Solid Edge part; units mm, degrees
sketch "Sketch1" plane through (0, 0, 0) normal (0, -1, 0) x (1, 0, 0)
  line L0 (2, 27.36) -> (2, 11.4867)
  line L1 (2, 11.4867) -> (4, 11.4867)
  line L2 (4, 11.4867) -> (4, 4.2309)
  line L3 (4, 4.2309) -> (7, 4.2309)
  line L4 (7, 4.2309) -> (7, 0)
  line L5 (7, 0) -> (1.25, 0)
  line L6 (1.25, 0) -> (1.25, 4.2309)
  line L7 (1.25, 27.36) -> (1.25, 4.2309)
  line L8 (1.25, 27.36) -> (2, 27.36)
revolve "RevolvedProtrusion1" add sketch "Sketch1" angle 360 about axis through (0, 0, 54) along (0, 0, -1)
cosmetic_thread "Thread1"
CAD build for the part. Positions are in the model's coordinates, mm. A direction names the side the tool comes from. Round coordinates to 2 decimals unless told otherwise and drop trailing zeros. Order: outer loops, then holes, each group sorted by start corner. A loop starts at its lowest first (then second) coordinate and runs counter-clockwise, first axis right, second up. Notation, with made-up numbers: (56.25, -1) -> (71.25, -1) arc R21 ccw to (71.25, 9) -> close; hole circle Ø8 at (-25.75, -33). An arc over 180 degrees is marked (long way). One line per question, with ' | ' between items.
Q1. Slice it at A-A (y = 0). Write the cut outline in (x, z), then the cut area to 3 significant figures.
Completed:
outline: (-7, 0) -> (-1.25, 0) -> (-1.25, 27.36) -> (-2, 27.36) -> (-2, 11.49) -> (-4, 11.49) -> (-4, 4.23) -> (-7, 4.23) -> close; (1.25, 0) -> (7, 0) -> (7, 4.23) -> (4, 4.23) -> (4, 11.49) -> (2, 11.49) -> (2, 27.36) -> (1.25, 27.36) -> close | area: 112 mm^2
Q2. Probe probe 1 along X at (y, z) = (0, 20.5); probe 2 along Y at (x, z) = (0, 7.75). List the from-to ranges inside material, lowest first.
Completed:
probe 1: x = -2 to -1.25, 1.25 to 2 | probe 2: y = -4 to -1.25, 1.25 to 4
Q3. Drop flat-ended pins along their axis: pin 1 (1 mm diameter, centred on y = 1.5, z = 16, fed in from -X); pin 2 (1.5 mm diameter, centred on x = 2.5, y = -2, fed in from +Z); pin 3 (5 mm diameter, centred on y = -5, z = 11.5, fed in from -X). Give the stop position or say it passes through.
Completed:
pin 1: stops at x = -1.73 | pin 2: stops at z = 11.49 | pin 3: stops at x = -3.12
Q4. Which spindle directions (+Z, -Z, +X, -X, +Y, -Y) get a long thin tool onto all of the face, cutting with end or side? Do faces 4 (the cylindrical face through (6.466, 2.681, 2.086)), 5 (the cylindrical face through (-0.867, 3.905, 7.808)). Say none if no direction does.
Completed:
face 4: +Z, -Z | face 5: +Z
Q5. Two-plate mould, pull along Y, no slides. Class faces 1 (the cylindrical face through (-0.27, -1.22, 13.87)), 2 (the cylindrical face through (0, 2, 19)), 3 (the flat face through (-0.1, 1.5, 0)): released by +Y, released by -Y, zero draft, split by the parting line, or undercut.
Completed:
face 1: undercut | face 2: split by the parting line | face 3: zero draft
Q6. Slice it at C-C (z = 12.75). Write the cut outline in (x, y).
Completed:
outline: circle Ø4 at (0, 0); hole circle Ø2.5 at (0, 0)
Q7. Slice it at D-D (x = 2.5). Write the cut outline in (y, z).
Completed:
outline: (-6.54, 0) -> (6.54, 0) -> (6.54, 4.23) -> (3.12, 4.23) -> (3.12, 11.49) -> (-3.12, 11.49) -> (-3.12, 4.23) -> (-6.54, 4.23) -> close
